Could you check a few things on this drawing? It's one solid part, dimensions in mm from its lowest x, y, z. A direction names the side the tool comes from. Round coordinates to 2 decimals unless told otherwise and drop trailing zeros. Loops run counter-clockwise (first coordinate to the right, second up) from the corner with the lowest first, then second, coordinate; pieces in that order, holes last. Notation, with made-up numbers: (20.5, 74.25) -> (75.5, 74.25) arc R22 ccw to (75.5, 83.25) -> close; hole circle Ø10 at (58.25, -4.75). An arc over 180 degrees is marked (long way). Put each result on its own line as item: value. Start each with the question number.
1. I'm going to push flat-ended pins straight in: P1, Ø2.5, axis at y = 5.5, z = 3, coming from the -X side; P2, Ø2, axis at x = 16, z = 3, coming from the +Y side; P3, Ø5, axis at x = 7, y = 5.5, coming from the +Z side. Where does each tip first touch, or does it pass through?
2. If we mould it in two halves opening along X, with no side actions, what happens to the marked faces 1, 2, 3 and 4? For each: pulls with the +X half, pulls with the -X half, needs draft (parallel to the pull), parting line crosses it, or undercut.
3. Imagine slicing it at D-D, the plane z = 0.8. Please give me the cut outline in (x, y) (1 decimal).
4. I need wall thicknesses on line 1 (X direction, y = 7, z = 0.4) (1 decimal); line 2 (Y direction, x = 18.75, z = 0.95); line 3 (Y direction, x = 24, z = 4.3) (1 decimal). Which ranges of each line are inside material? Lowest first, please. Write a range as [from, to].
5. Which directions (+Z, -Z, +X, -X, +Y, -Y) give clear straight access to the entire face, cutting with the end or side of a thin tool? Please do the marked faces 5 and 6.
6. Imagine slicing it at C-C, the plane x = 15.5. Please give me the cut outline in (y, z).
7. Imagine slicing it at B-B, the plane z = 3.3. Please give me the cut outline in (x, y) (1 decimal).
8. Imagine slicing it at A-A, the plane y = 2.75. Please give me the cut outline in (x, z) (1 decimal), and give its area (3 significant figures).
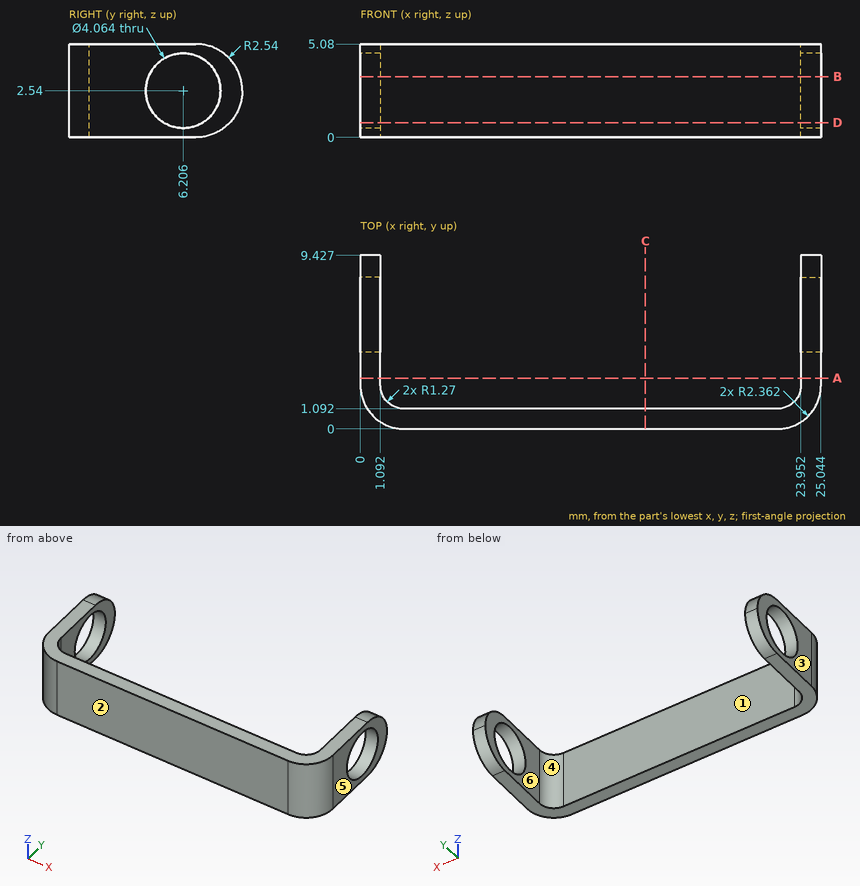
Entries:
1. P1: x = 0
1. P2: y = 1.09
1. P3: through
2. face 1: undercut
2. face 2: needs draft
2. face 3: pulls with the -X half
2. face 4: undercut
3. outline: (0, 2.4) arc R2.4 ccw to (2.4, 0) -> (22.7, 0) arc R2.4 ccw to (25, 2.4) -> (25, 5.2) -> (24, 5.2) -> (24, 2.4) arc R1.3 cw to (22.7, 1.1) -> (2.4, 1.1) arc R1.3 cw to (1.1, 2.4) -> (1.1, 5.2) -> (0, 5.2) -> close; (0, 7.3) -> (1.1, 7.3) -> (1.1, 8.7) -> (0, 8.7) -> close; (24, 7.3) -> (25, 7.3) -> (25, 8.7) -> (24, 8.7) -> close
4. line 1: [0, 1.1], [24, 25]
4. line 2: [0, 1.09]
4. line 3: [0.4, 5.2], [7.2, 8.7]
5. face 5: +Z, -Z, +X, +Y, -Y
5. face 6: +Z, -Z, +Y
6. outline: (0, 0) -> (1.09, 0) -> (1.09, 5.08) -> (0, 5.08) -> close
7. outline: (0, 2.4) arc R2.4 ccw to (2.4, 0) -> (22.7, 0) arc R2.4 ccw to (25, 2.4) -> (25, 4.3) -> (24, 4.3) -> (24, 2.4) arc R1.3 cw to (22.7, 1.1) -> (2.4, 1.1) arc R1.3 cw to (1.1, 2.4) -> (1.1, 4.3) -> (0, 4.3) -> close; (0, 8.1) -> (1.1, 8.1) -> (1.1, 9.3) -> (0, 9.3) -> close; (24, 8.1) -> (25, 8.1) -> (25, 9.3) -> (24, 9.3) -> close
8. outline: (0, 0) -> (1.1, 0) -> (1.1, 5.1) -> (0, 5.1) -> close; (24, 0) -> (25, 0) -> (25, 5.1) -> (24, 5.1) -> close
8. area: 11.1 mm^2
